from build123d import *

# Parameters (mm, degrees)
BOSS_EXTRUDE1_DEPTH = 5
CUT_EXTRUDE1_DEPTH  = 5
SKETCH10_R          = 4
SKETCH10_R_2        = 2
BOSS_EXTRUDE3_DEPTH = 5
SKETCH11_R          = 2
CUT_EXTRUDE3_DEPTH  = 5


with BuildPart() as part:
    # Sketch1 → Boss-Extrude1 (new body)
    with BuildSketch(Plane.XY):
        Polygon((7.5, 32.5), (7.5, 37.5), (-7.5, 37.5), (-7.5, 32.5), (-30, 32.5), (-30, 10), (-35, 10), (-35, -10), (-30, -10), (-30, -32.5), (30, -32.5), (30, 32.5), align=None)
    extrude(amount=BOSS_EXTRUDE1_DEPTH)

    # Sketch3 → Cut-Extrude1 (cut)
    with BuildSketch(Plane.XY.offset(5)):
        Polygon((30, 24.5), (25, 24.5), (25, 26), (21.6, 26), (21.6, 24.5), (10, 24.5), (10, 20.1), (21.6, 20.1), (21.6, 18.6), (25, 18.6), (25, 20.1), (30, 20.1), align=None)
        Polygon((30, -24.5), (30, -20.1), (25, -20.1), (25, -18.6), (21.6, -18.6), (21.6, -20.1), (10, -20.1), (10, -24.5), (21.6, -24.5), (21.6, -26), (25, -26), (25, -24.5), align=None)
        Polygon((-30, -24.5), (-25, -24.5), (-25, -26), (-21.6, -26), (-21.6, -24.5), (-10, -24.5), (-10, -20.1), (-21.6, -20.1), (-21.6, -18.6), (-25, -18.6), (-25, -20.1), (-30, -20.1), align=None)
    extrude(amount=-CUT_EXTRUDE1_DEPTH, mode=Mode.SUBTRACT)

    # Sketch10 → Boss-Extrude3 (add)
    with BuildSketch(Plane.XY.offset(5)):
        with Locations((0, -32.5)):
            Circle(SKETCH10_R)
        with Locations((0, -32.5)):
            Circle(SKETCH10_R_2, mode=Mode.SUBTRACT)
    extrude(amount=-BOSS_EXTRUDE3_DEPTH)

    # Sketch11 → Cut-Extrude3 (cut)
    with BuildSketch(Plane.XY.offset(5)):
        with Locations((0, -32.5)):
            Circle(SKETCH11_R)
    extrude(amount=-CUT_EXTRUDE3_DEPTH, mode=Mode.SUBTRACT)


solid = part.part
Check sheet for the modelled part. Datum: model origin and axes. Units: mm. A direction names the side the tool comes from. Round coordinates to 2 decimals unless told otherwise and drop trailing zeros. Order: outer loops, then holes, each group sorted by start corner. A loop starts at its lowest first (then second) coordinate and runs counter-clockwise, first axis right, second up.
Q1. Cross-section at A-A, the plane x = 0. Enter the section's corners in (y, z).
Filled sheet:
outline: (-36.5, 0) - (-34.5, 0) - (-34.5, 5) - (-36.5, 5) - close; (-30.5, 0) - (37.5, 0) - (37.5, 5) - (-30.5, 5) - close
Q2. Scan lines: L1, parallel to Y at x = 0, z = 2.1; L2, parallel to Y at x = 15, z = 0.25; L3, parallel to Y at x = -13, z = 3.85. Record each from-to range of solid material in increasing order.
Filled sheet:
L1: y = -36.5 to -34.5, -30.5 to 37.5
L2: y = -32.5 to -24.5, -20.1 to 20.1, 24.5 to 32.5
L3: y = -32.5 to -24.5, -20.1 to 32.5
Q3. Depth check by flat-ended pin: P1, Ø2.5, axis at x = 14.5, z = 2.5, coming from the -Y side; P2, Ø2, axis at y = 17.5, z = 2.5, coming from the -X side; P3, Ø2.5, axis at x = 0, y = -32.5, coming from the +Z side; P4, Ø2.5, axis at x = 15, z = 2, coming from the +Y side. Enter the tip coordinate at first touch or a pass-through.
Filled sheet:
P1: stops at y = -32.5
P2: stops at x = -30
P3: passes through
P4: stops at y = 32.5
Q4. Draft check along Y on faces 1 (the face through (-3, 1, 0)), 2 (the face through (-23, -26, 3)), 3 (the face through (-33, -10, 2)). Enter one of: pulls with the +Y half, pulls with the -Y half, needs draft (parallel to the pull), parting line crosses it, or undercut.
Filled sheet:
face 1: needs draft
face 2: undercut
face 3: pulls with the -Y half
Q5. Cross-section at D-D, the plane x = -23.5. Enter the section's corners in (y, z), plus the area to 3 significant figures.
Filled sheet:
outline: (-32.5, 0) - (-26, 0) - (-26, 5) - (-32.5, 5) - close; (-18.6, 0) - (32.5, 0) - (32.5, 5) - (-18.6, 5) - close
area: 288 mm2
Q6. Cross-section at B-B, the plane x = 13. Enter the section's corners in (y, z), plus the area to 3 significant figures.
Filled sheet:
outline: (-32.5, 0) - (-24.5, 0) - (-24.5, 5) - (-32.5, 5) - close; (-20.1, 0) - (20.1, 0) - (20.1, 5) - (-20.1, 5) - close; (24.5, 0) - (32.5, 0) - (32.5, 5) - (24.5, 5) - close
area: 281 mm2
Q7. Cross-section at C-C, the plane y = -28. Enter the section's corners in (x, z), plus the area to 3 significant figures.
Filled sheet:
outline: (-30, 0) - (30, 0) - (30, 5) - (-30, 5) - close
area: 300 mm2
Q8. Set-up check for faces 4 (the face through (-16, -24.5, 3)), 5 (the face through (27, 20.1, 3)), 6 (the face through (23, -18.6, 3)): record each of +Z, -Z, +X, -X, +Y, -Y from which the full face is reachable in a straight line by a thin tool's end or side.
Filled sheet:
face 4: +Z, -Z, -X
face 5: +Z, -Z, +X
face 6: +Z, -Z
